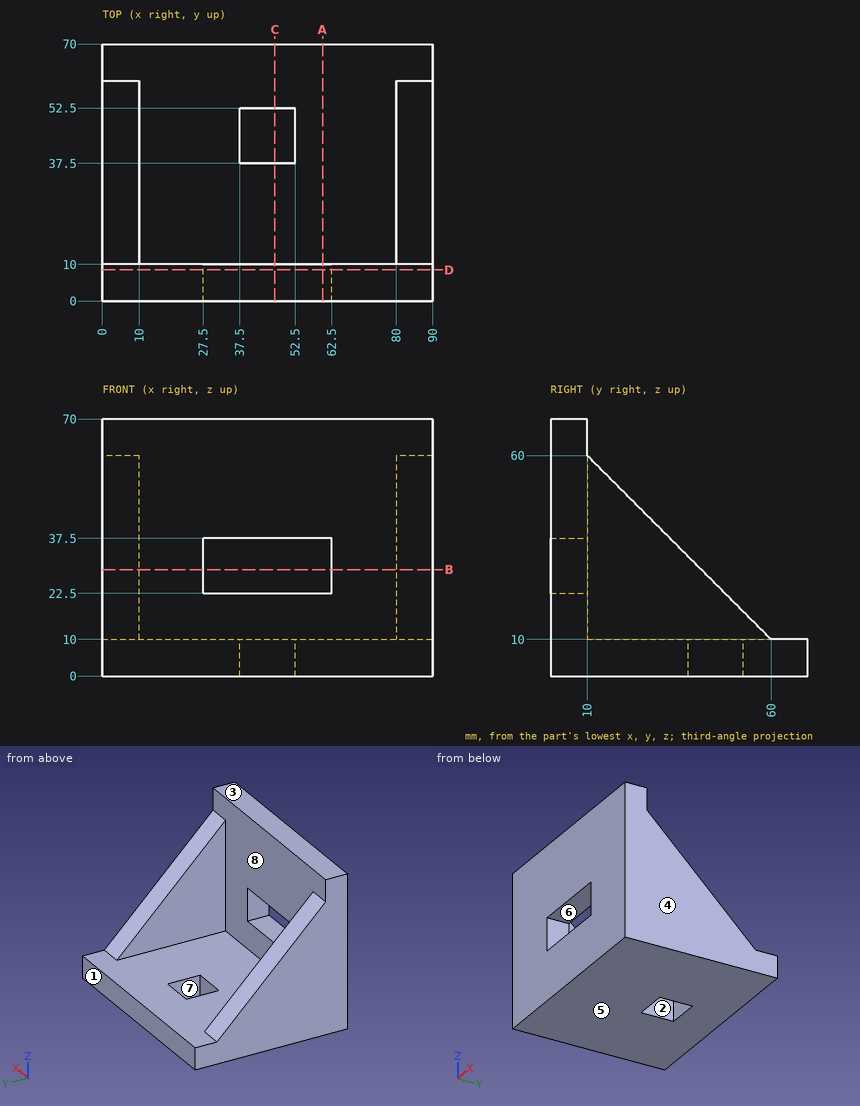
Geometry: see drawing. Coordinates: mm, zero at the bounding-box minimum. A direction names the side the tool comes from. Give positions to 0.01 mm unless a question says otherwise; leave off trailing zeros. Write each loop counter-clockwise with the first axis right and the second up, starting at its lowest first coordinate (ties: lowest second). Pieces come first, ordered by that corner, then holes. Notation, with made-up numbers: M 23,23 L 32,23 A18 cw 32,33 Z; hole C 47.25,80 d8. An arc over 180 degrees is marked long. Answer in a Markdown table with one row per item. Add a question column.
(1) Mould query, pull axis Y, two halves, no side actions, for the marked faces 1, 2 and 3. Classes: +Y half, -Y half, draft (parallel to the pull), parting line (faces both ways), or undercut.
(2) Section B-B on z = 29. Return loops of the section in (x, y).
(3) Section C-C on x = 47. Return loops of the section in (y, z), and give its area (3 significant figures).
(4) Section A-A on x = 60. Return loops of the section in (y, z), and give its area (3 significant figures).
(5) Ray query, line 1 (Y direction, x = 34, z = 52); line 2 (X direction, y = 45, z = 8). Return the intervals inside material, ascending.
(6) Section D-D on y = 8.5. Return loops of the section in (x, z).
(7) First-contact query: pin 1 (3 mm diameter, centred on x = 76.5, y = 48, fed in from -Z); pin 2 (8 mm diameter, centred on x = 11, z = 47.5, fed in from +Y); pin 3 (4 mm diameter, centred on x = 14, y = 32.5, fed in from +Z); pin 4 (18 mm diameter, centred on x = 51, z = 36.5, fed in from +Y). Flat tips, straight axial feed; report the tip coordinate or a pass-through.
(8) Reachability of the marked faces 4, 5, 6, 7 and 8 from +Z, -Z, +X, -X, +Y, -Y: full face, straight path, thin tool, end or side. Return the list, or none.
Result set:
| question | item | result |
|---|---|---|
| 1 | face 1 | +Y half |
| 1 | face 2 | undercut |
| 1 | face 3 | draft |
| 2 | outline | M 0,0 L 27.5,0 L 27.5,10 L 10,10 L 10,41 L 0,41 Z; M 62.5,0 L 90,0 L 90,41 L 80,41 L 80,10 L 62.5,10 Z |
| 3 | outline | M 0,0 L 37.5,0 L 37.5,10 L 10,10 L 10,22.5 L 0,22.5 Z; M 0,37.5 L 10,37.5 L 10,70 L 0,70 Z; M 52.5,0 L 70,0 L 70,10 L 52.5,10 Z |
| 3 | area | 1,000 mm^2 |
| 4 | outline | M 0,0 L 70,0 L 70,10 L 10,10 L 10,22.5 L 0,22.5 Z; M 0,37.5 L 10,37.5 L 10,70 L 0,70 Z |
| 4 | area | 1,150 mm^2 |
| 5 | line 1 | y = 0 to 10 |
| 5 | line 2 | x = 0 to 37.5, 52.5 to 90 |
| 6 | outline | M 0,0 L 90,0 L 90,70 L 0,70 Z; hole M 27.5,22.5 L 62.5,22.5 L 62.5,37.5 L 27.5,37.5 Z |
| 7 | pin 1 | stops at z = 0 |
| 7 | pin 2 | stops at y = 26.37 |
| 7 | pin 3 | stops at z = 10 |
| 7 | pin 4 | stops at y = 10 |
| 8 | face 4 | +Z, -Z, +X, +Y, -Y |
| 8 | face 5 | -Z, +X, -X, +Y, -Y |
| 8 | face 6 | +Y, -Y |
| 8 | face 7 | +Z, -Z |
| 8 | face 8 | +Z, +Y |
